For this review, take the finished solid that the model builds, in its own axes (mm). Coordinates: 2 decimals unless noted, no trailing zeros. Loops run counter-clockwise (first coordinate to the right, second up) from the corner with the lowest first, then second, coordinate; pieces in that order, holes last. Notation, with made-up numbers: M 1.5,-26.5 L 20.5,-26.5 A16 ccw 20.5,-3.5 Z; hole C 81,61.25 d10. An arc over 180 degrees is marked long. Use one line per item in the form item = value.
Autodesk Inventor part; units mm, degrees
ref_plane "YZ Plane" through (0, 0, 0) normal (1, 0, 0) x (0, 1, 0)
ref_plane "XZ Plane" through (0, 0, 0) normal (0, 1, 0) x (-1, 0, 0)
ref_plane "XY Plane" through (0, 0, 0) normal (0, 0, 1) x (1, 0, 0)
sketch "Sketch1" plane through (0, 0, 0) normal (1, 0, 0) x (0, 1, 0)
  line L0 (3.2881, 15.1027) -> (-1.2119, 15.1027)
  line L1 (-1.2119, 15.1027) -> (-1.2119, -2.8973)
  line L2 (-1.2119, -2.8973) -> (3.2881, -2.8973)
  line L3 (3.2881, -2.8973) -> (3.2881, 15.1027)
  point P0 (0, 0)
  dimension "d0" = 4.5
  dimension "d1" = 18
extrude "Extrusion1" add sketch "Sketch1" along normal blind 21
sketch "Sketch2" plane through (0, 3.2881, 15.1027) normal (0, 1, 0) x (1, 0, 0)
  circle A0 centre (10.5, 3) radius 2
  circle A1 centre (10.5, 3) radius 2
  circle A2 centre (10.5, 15) radius 2
  line L0 (0, 18) -> (21, 18)
  line L1 (0, 0) -> (21, 0)
  line L2 (0, 18) -> (0, 0)
  point P0 (0, 15.1027)
  dimension "d4" = 18
  dimension "d5" = 12
  dimension "d6" = 3
  dimension "d7" = 10.5
  dimension "d8" = 21
  dimension "d9" = 10.5
sketch "Sketch3" plane through (0, -1.2119, -2.8973) normal (0, 0, -1) x (-1, 0, 0)
  circle A0 centre (-4.5, 2.25) radius 2
  circle A1 centre (-4.5, 2.25) radius 2
  circle A2 centre (-16.5, 2.25) radius 2
  line L0 (0, 4.5) -> (-21, 4.5)
  line L1 (0, 0) -> (0, 4.5)
  point P0 (0, 1.2119)
  dimension "d10" = 12
  dimension "d11" = 2.25
  dimension "d12" = 2.25
  dimension "d13" = 4.5
extrude "Extrusion2" cut sketch "Sketch2" against normal through all
extrude "Extrusion3" cut sketch "Sketch3" against normal through all
equation "\"d7\" = 0.5 * d8"
equation "\"d9\" = d7"
equation "\"d12\" = d11"
properties part number "XL_XL_interface_v2"
1. Consider section B-B on y = -0.05. Write out the cut boundary in (x, z).
Computed values:
outline = M 0,-2.9 L 2.82,-2.9 L 2.82,15.1 L 0,15.1 Z; M 6.18,-2.9 L 14.82,-2.9 L 14.82,15.1 L 6.18,15.1 Z; M 18.18,-2.9 L 21,-2.9 L 21,15.1 L 18.18,15.1 Z; hole C 10.5,0.1 d4; hole C 10.5,12.1 d4
2. Wall thickness on line 1 along Z through (x, y) = (10.5, 0.2); line 2 along X through (y, z) = (0.95, 9.5); line 3 along X through (y, z) = (-0.25, 6.75): over which ranges is each line inside the solid? List them lowest first. Write a range as from..to.
Computed values:
line_1 = -2.9..-1.9, 2.1..10.1, 14.1..15.1
line_2 = 0..2.5, 6.5..14.5, 18.5..21
line_3 = 0..2.97, 6.03..14.97, 18.03..21
3. Consider section D-D on z = 10.5. Write out the cut boundary in (x, y).
Computed values:
outline = M 0,-1.21 L 9.3,-1.21 L 9.3,3.29 L 0,3.29 Z; M 11.7,-1.21 L 21,-1.21 L 21,3.29 L 11.7,3.29 Z; hole C 4.5,1.04 d4; hole C 16.5,1.04 d4
4. Consider section C-C on x = 4.5. Write out the cut boundary in (y, z).
Computed values:
outline = M -1.21,-2.9 L -0.96,-2.9 L -0.96,15.1 L -1.21,15.1 Z; M 3.04,-2.9 L 3.29,-2.9 L 3.29,15.1 L 3.04,15.1 Z
5. Draft analysis for pull direction Z (two halves, no side actions). For faces 1 (the face through (10, 1, -2.897)), 2 (the face through (10.066, 1.07, 14.055)), 3 (the face through (10, -1.212, 6)), state which applies: +Z half, -Z half, draft (parallel to the pull), parting line (faces both ways), or undercut.
Computed values:
face_1 = -Z half
face_2 = undercut
face_3 = draft
6. Consider section A-A on x = 10.5. Write out the cut boundary in (y, z).
Computed values:
outline = M -1.21,-2.9 L 3.29,-2.9 L 3.29,-1.9 L -1.21,-1.9 Z; M -1.21,2.1 L 3.29,2.1 L 3.29,10.1 L -1.21,10.1 Z; M -1.21,14.1 L 3.29,14.1 L 3.29,15.1 L -1.21,15.1 Z
